Design review of the part built by this model. Coordinates are the model's own, in mm. Face numbers are marked on the shaded views. A direction names the side the tool comes from. Coordinates: 2 decimals unless noted, no trailing zeros. Loops run counter-clockwise (first coordinate to the right, second up) from the corner with the lowest first, then second, coordinate; pieces in that order, holes last. Notation, with made-up numbers: (11.25, 60.25) - (31.25, 60.25) arc R19 ccw to (31.25, 92.25) - close; hole circle Ø5 at (71, 63). An arc over 180 degrees is marked (long way). Use one line per item in the form item = value. Start each with the question number.
(1) Add section C-C (y = 37). Count the separate pieces of the cut face and the enclosed holes in it, plus the area to 3 significant figures.
(2) For L1, parallel to X at y = 38.25, z = 3; L2, parallel to Z at x = -28.1, y = 36.25; L3, parallel to Y at x = -7, z = 1.5, list the stretches that pass through material, from the lowest coordinate up.
(3) Add section D-D (z = 6.5). State the section outline as (x, y) points.
(4) Clearance check with flat-ended pins moving along their axes: pin 1 Ø1.6 at (y, z) = (36.5, 3.5) entering from -X; pin 2 Ø1.9 at (x, y) = (-15, 36.25) entering from -Z; pin 3 Ø1.9 at (y, z) = (36.25, 3.5) entering from +X. State where each tip first meets the part, or that it passes through.
(5) Add section B-B (z = 3.5). State the section outline as (x, y) points, plus the area to 3 significant figures.
(6) Add section A-A (x = -7). State the section outline as (y, z) points, plus the area to 3 significant figures.
(7) The part is to be moulded in two halves that separate along X. For the marked faces 3, 4 and 5, say which applies: pulls with the +X half, pulls with the -X half, needs draft (parallel to the pull), parting line crosses it, or undercut.
(8) Tool access review of the marked faces 1 and 2: name each direction out of +Z, -Z, +X, -X, +Y, -Y from which nothing blocks a thin tool from reaching the whole face with its end or side.
```python
from build123d import *

# Parameters (mm, degrees)
SKETCH1_W                      = 27
SKETCH1_H                      = 7
BOSS_EXTRUDE1_DEPTH            = 7
SIDE_SHAFT_HOLES_M3_AT_2_COUNT = 2
SIDE_SHAFT_HOLES_M3_AT_2_PITCH = 48.812875198
SKETCH9_R                      = 1.6
BOSS_EXTRUDE2_DEPTH            = 3.4
M3_CLEARANCE_HOLE1_D           = 3.2
CUT_EXTRUDE1_START             = -2.1
CUT_EXTRUDE1_DEPTH             = 2.6


with BuildPart() as part:
    # Sketch1 → Boss-Extrude1 (new body)
    with BuildSketch(Plane.XY):
        with Locations((-15, 36.25)):
            Rectangle(SKETCH1_W, SKETCH1_H)
    extrude(amount=BOSS_EXTRUDE1_DEPTH)

    # Sketch2 → Side Shaft Holes (M3) (revolve, cut)
    with BuildSketch(Plane(origin=(-1.5, 36.25, 3.5), x_dir=(0, 0, -1), z_dir=(0, 1, 0))):
        Polygon((0, 0), (0, 4), (1.6, 3.03862301), (1.6, 0), align=None)
    side_shaft_holes_m3 = revolve(axis=Axis((4.85, 36.25, 3.5), (-1, 0, 0)), mode=Mode.SUBTRACT)

    # Side Shaft Holes (M3) at 2: Side Shaft Holes (M3) ×2
    with Locations(*[(0, 0, -i * SIDE_SHAFT_HOLES_M3_AT_2_PITCH) for i in range(1, SIDE_SHAFT_HOLES_M3_AT_2_COUNT)]):
        add(side_shaft_holes_m3, mode=Mode.SUBTRACT)

    # Sketch9 → Boss-Extrude2 (add)
    with BuildSketch(Plane.ZY.offset(4.53862301)):
        with Locations(Location((3.5, 36.25, 0), (0, 0, 180))):
            Circle(SKETCH9_R)
    boss_extrude2 = extrude(amount=BOSS_EXTRUDE2_DEPTH)

    # Shaft Hole Mirror: Side Shaft Holes (M3), Boss-Extrude2 across plane
    add(side_shaft_holes_m3.mirror(Plane.ZY.offset(15)), mode=Mode.SUBTRACT)
    add(boss_extrude2.mirror(Plane.ZY.offset(15)))

    # Shaft Hole Mirror copy 1 sketch → Shaft Hole Mirror copy 1 (revolve, cut)
    with BuildSketch(Plane(origin=(-28.5, 36.25, -45.312875198), x_dir=(0, 0, -1), z_dir=(0, 1, 0))):
        Polygon((0, 0), (0, -4), (1.6, -3.03862301), (1.6, 0), align=None)
    revolve(axis=Axis((-34.85, 36.25, -45.312875198), (-1, 0, 0)), mode=Mode.SUBTRACT)

    # M3 Clearance Hole1 (through all)
    with Locations(Plane.XY.offset(7)):
        with Locations((-7, 36.25), (-15, 36.25), (-23, 36.25)):
            Hole(M3_CLEARANCE_HOLE1_D / 2)

    # Sketch8 → Cut-Extrude1 (cut)
    with BuildSketch(Plane.ZY.offset(4.53862301).offset(CUT_EXTRUDE1_START)):
        Polygon((0.324573519, 36.25), (1.91228676, 33.5), (5.08771324, 33.5), (7, 33.5), (7, 39), (5.08771324, 39), (1.91228676, 39), align=None)
    cut_extrude1 = extrude(amount=CUT_EXTRUDE1_DEPTH, mode=Mode.SUBTRACT)

    # Mirror1: Cut-Extrude1 across plane
    add(cut_extrude1.mirror(Plane.ZY.offset(15)), mode=Mode.SUBTRACT)


solid = part.part
```
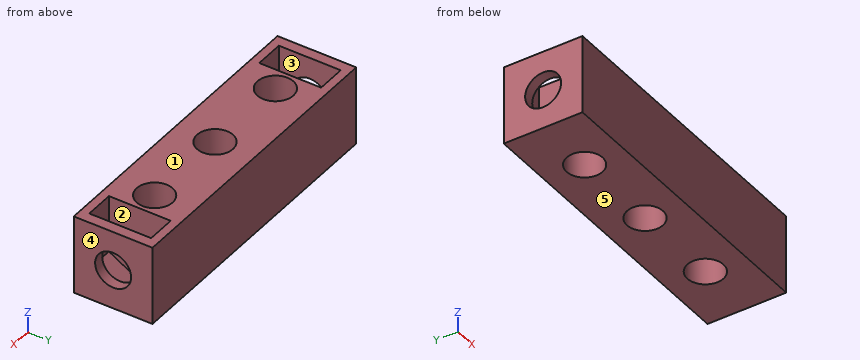
Computed values:
q1.separate_pieces = 6
q1.enclosed_holes = 0
q1.area = 91.9 mm^2
q2.L1 = -28.5 to -27.56, -24.96 to -5.04, -2.44 to -1.5
q2.L2 = 0 to 1.9, 5.1 to 7
q2.L3 = 32.75 to 34.65, 37.85 to 39.75
q3.outline = (-28.5, 32.75) - (-1.5, 32.75) - (-1.5, 39.75) - (-28.5, 39.75) - close; hole (-27.56, 33.5) - (-24.96, 33.5) - (-24.96, 39) - (-27.56, 39) - close; hole circle Ø3.2 at (-23, 36.25); hole circle Ø3.2 at (-15, 36.25); hole circle Ø3.2 at (-7, 36.25); hole (-5.04, 33.5) - (-2.44, 33.5) - (-2.44, 39) - (-5.04, 39) - close
q4.pin_1 = -24.96
q4.pin_2 = through
q4.pin_3 = -5.04
q5.outline = (-28.5, 32.75) - (-1.5, 32.75) - (-1.5, 34.65) - (-2.44, 34.65) - (-2.44, 33.5) - (-5.04, 33.5) - (-5.04, 39) - (-2.44, 39) - (-2.44, 37.85) - (-1.5, 37.85) - (-1.5, 39.75) - (-28.5, 39.75) - (-28.5, 37.85) - (-27.56, 37.85) - (-27.56, 39) - (-24.96, 39) - (-24.96, 33.5) - (-27.56, 33.5) - (-27.56, 34.65) - (-28.5, 34.65) - close; hole circle Ø3.2 at (-23, 36.25); hole circle Ø3.2 at (-15, 36.25); hole circle Ø3.2 at (-7, 36.25)
q5.area = 130 mm^2
q6.outline = (32.75, 0) - (34.65, 0) - (34.65, 7) - (32.75, 7) - close; (37.85, 0) - (39.75, 0) - (39.75, 7) - (37.85, 7) - close
q6.area = 26.6 mm^2
q7.face_3 = undercut
q7.face_4 = pulls with the +X half
q7.face_5 = needs draft
q8.face_1 = +Z, +X, -X, +Y, -Y
q8.face_2 = +Z
